For this review, take the finished solid that the model builds, in its own axes (mm). Face numbers are marked on the shaded views. A direction names the side the tool comes from. Coordinates: 2 decimals unless noted, no trailing zeros. Order: outer loops, then holes, each group sorted by start corner. A loop starts at its lowest first (then second) coordinate and runs counter-clockwise, first axis right, second up.
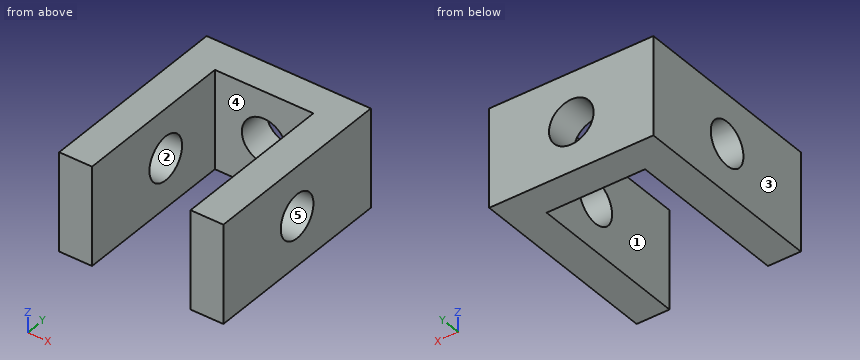
Solid Edge part; units mm, degrees
sketch "Sketch1" plane through (0, 0, 0) normal (0, -1, 0) x (1, 0, 0)
  line L0 (0, 0) -> (25, 0)
  line L1 (25, 0) -> (25, 15)
  line L2 (25, 15) -> (0, 15)
  line L3 (0, 15) -> (0, 0)
extrude "Protrusion1" add sketch "Sketch1" against normal blind 30
shell "Thinwall_1" thickness 5 removed faces 3 at (4.4167, 0, 12.65) at (21.0833, 24.7, 15) at (3.9167, 24.7, 0)
hole "Hole_1" at (25, 15, 7.5) direction (-1, 0, 0) diameter 6.647 end up to next thread major 8 thread length 50.8
hole "M8_holes" at (0, 15, 7.5) direction (1, 0, 0) diameter 6.647 end up to next thread major 8 thread length 50.8
hole "Hole_3" at (12.5, 30, 7.5) direction (0, -1, 0) diameter 6.792 end up to next
1. The part is to be moulded in two halves that separate along X. For the marked faces 1, 2 and 3, say which applies: +X half, -X half, draft (parallel to the pull), parting line (faces both ways), or undercut.
Answer below:
face 1: undercut
face 2: draft
face 3: -X half
2. Take a section at B-B, the plane x = 12.5. Give the boundary of the cut face in (y, z), plus the area to 3 significant figures.
Answer below:
outline: (25, 0) - (30, 0) - (30, 4.1) - (25, 4.1) - close; (25, 10.9) - (30, 10.9) - (30, 15) - (25, 15) - close
area: 41.0 mm2
3. Machinability: for the marked faces 4 and 5, which of the approach directions +Z, -Z, +X, -X, +Y, -Y give a long, thin tool a straight path to every point of the face, cutting with its end or side? Answer none if there is none.
Answer below:
face 4: +Z, -Z, -Y
face 5: +X, -X
4. Take a section at A-A, the plane y = 15. Give the boundary of the cut face in (x, z), plus the area to 3 significant figures.
Answer below:
outline: (0, 0) - (5, 0) - (5, 4.18) - (0, 4.18) - close; (0, 10.82) - (5, 10.82) - (5, 15) - (0, 15) - close; (20, 0) - (25, 0) - (25, 4.18) - (20, 4.18) - close; (20, 10.82) - (25, 10.82) - (25, 15) - (20, 15) - close
area: 83.5 mm2
5. Take a section at D-D, the plane y = 8.25. Give the boundary of the cut face in (x, z).
Answer below:
outline: (0, 0) - (5, 0) - (5, 15) - (0, 15) - close; (20, 0) - (25, 0) - (25, 15) - (20, 15) - close
6. Clearance check with flat-ended pins moving along their axes: pin 1 Ø6 at (y, z) = (15, 7.5) entering from -X; pin 2 Ø4 at (x, z) = (16.5, 2) entering from -Y. State where each tip first meets the part, or that it passes through.
Answer below:
pin 1: passes through
pin 2: stops at y = 25
7. Take a section at C-C, the plane z = 7.5. Give the boundary of the cut face in (x, y), plus the area to 3 significant figures.
Answer below:
outline: (0, 0) - (5, 0) - (5, 11.68) - (0, 11.68) - close; (0, 18.32) - (5, 18.32) - (5, 25) - (9.1, 25) - (9.1, 30) - (0, 30) - close; (15.9, 25) - (20, 25) - (20, 18.32) - (25, 18.32) - (25, 30) - (15.9, 30) - close; (20, 0) - (25, 0) - (25, 11.68) - (20, 11.68) - close
area: 275 mm2
8. To check wall thickness, follow L1, parallel to X at y = 16, z = 12.25; L2, parallel to Y at x = 3, z = 7.5; L3, parallel to Z at x = 3.35, y = 15. State the ranges of each line that lie inside material, in increasing order.
Answer below:
L1: x = 0 to 5, 20 to 25
L2: y = 0 to 11.68, 18.32 to 30
L3: z = 0 to 4.18, 10.82 to 15
